from build123d import *

# Parameters (mm, degrees)
SKETCH1_R           = 3.302
BOSS_EXTRUDE1_DEPTH = 6.35
BOSS_EXTRUDE2_START = -6.35
SKETCH2_R           = 3.302
BOSS_EXTRUDE2_DEPTH = 1.5875
BOSS_EXTRUDE3_DEPTH = 12.7
FILLET1_R           = 1.5875
FILLET2_R           = 1.5875


with BuildPart() as part:
    # Sketch1 → Boss-Extrude1 (new body)
    with BuildSketch(Plane.XY):
        with BuildLine():
            Line((10.31875, 31.75), (10.31875, 0))
            ThreePointArc((10.31875, 0), (0, -10.31875), (-10.31875, 0))
            Line((-10.31875, 0), (-10.31875, 31.75))
            ThreePointArc((-10.31875, 31.75), (0, 42.06875), (10.31875, 31.75))
        make_face()
        Circle(SKETCH1_R, mode=Mode.SUBTRACT)
        with Locations((0, 31.75)):
            Circle(SKETCH1_R, mode=Mode.SUBTRACT)
    extrude(amount=BOSS_EXTRUDE1_DEPTH)

    # Sketch2 → Boss-Extrude2 (add)
    with BuildSketch(Plane(origin=(0, 0, 0), x_dir=(-1, 0, 0), z_dir=(0, 0, -1)).offset(BOSS_EXTRUDE2_START)):
        with BuildLine():
            Line((-23.31351417, 8.06700825), (-13.502035234, 36.4220125))
            ThreePointArc((-13.502035234, 36.4220125), (0, 46.0375), (13.502035234, 36.4220125))
            Line((13.502035234, 36.4220125), (23.31351417, 8.06700825))
            ThreePointArc((23.31351417, 8.06700825), (0, -24.66975), (-23.31351417, 8.06700825))
        make_face()
        Circle(SKETCH2_R, mode=Mode.SUBTRACT)
        with Locations((0, 31.75)):
            Circle(SKETCH2_R, mode=Mode.SUBTRACT)
    extrude(amount=BOSS_EXTRUDE2_DEPTH)

    # Sketch3 → Boss-Extrude3 (add)
    with BuildSketch(Plane.XY.offset(6.35)):
        with BuildLine():
            Line((-13.502035234, 36.4220125), (-23.31351417, 8.06700825))
            ThreePointArc((-23.31351417, 8.06700825), (0, -24.66975), (23.31351417, 8.06700825))
            Line((23.31351417, 8.06700825), (13.502035234, 36.4220125))
            ThreePointArc((13.502035234, 36.4220125), (0, 46.0375), (-13.502035234, 36.4220125))
        make_face()
        with BuildLine():
            Line((21.813288033, 7.54789575), (12.001809097, 35.9029))
            ThreePointArc((12.001809097, 35.9029), (0, 44.45), (-12.001809097, 35.9029))
            Line((-12.001809097, 35.9029), (-21.813288033, 7.54789575))
            ThreePointArc((-21.813288033, 7.54789575), (0, -23.08225), (21.813288033, 7.54789575))
        make_face(mode=Mode.SUBTRACT)
    extrude(amount=BOSS_EXTRUDE3_DEPTH)

    # Fillet1
    fillet1_edges = [part.edges().sort_by_distance(p)[0] for p in [
        (10.31875, 15.875, 4.7625),
        (0, 42.06875, 4.7625),
        (-10.31875, 15.875, 4.7625),
        (0, -10.31875, 4.7625),
        (0, 46.0375, 4.7625),
        (18.407774702, 22.244510375, 4.7625),
        (0, -24.66975, 4.7625),
        (-18.407774702, 22.244510375, 4.7625),
        (0, -23.08225, 6.35),
        (16.907548565, 21.725397875, 6.35),
        (0, 44.45, 6.35),
        (-16.907548565, 21.725397875, 6.35),
    ]]
    fillet(fillet1_edges, radius=FILLET1_R)

    # Fillet2
    fillet2_edges = [part.edges().sort_by_distance(p)[0] for p in [
        (10.31875, 15.875, 0),
        (0, -10.31875, 0),
        (-10.31875, 15.875, 0),
        (0, 42.06875, 0),
    ]]
    fillet(fillet2_edges, radius=FILLET2_R)


solid = part.part
Geometry: final body of the model. Coordinates: model frame, mm. A direction names the side the tool comes from. Give positions to 0.01 mm unless a question says otherwise; leave off trailing zeros.
(1) First-contact query: P1, Ø7.5, axis at x = 0, y = 31.75, coming from the +Z side; P2, Ø5.5, axis at x = 0, y = 0, coming from the -Z side; P3, Ø8, axis at x = -10.5, y = 19.5, coming from the -Z side; P4, Ø1.7, axis at y = 16, z = 2.5, coming from the +X side. Flat tips, straight axial feed; report the tip coordinate or a pass-through.
(2) Access query for faces 1 (the cylindrical face through (0.227, -10.316, 2.37)), 2 (the flat face through (10.319, 16, 2)), 3 (the cylindrical face through (17.89, 22.29, 5.22)), 4 (the flat face through (16.976, 21.527, 13.416)). Directions: +Z, -Z, +X, -X, +Y, -Y. A direction counts if a zero-diameter tool reaches every point of the face in a straight line with its end or side. Return the directions, or none.
(3) Ray query, line 1 (Y direction, x = 0, z = 2.25); line 2 (X direction, y = -0.5, z = 17.5); line 3 (Y direction, x = 0, z = 16). Return the intervals inside material, ascending.
(4) Mould query, pull axis Y, two halves, no side actions, for faces 5 (the flat face through (-12, -2, 4.762)), 6 (the flat face through (0, 11, 6.35)), 7 (the flat face through (18.476, 22.046, 12.611)). Classes: released by +Y, released by -Y, zero draft, split by the parting line, or undercut.
(5) Cut plane A-A, the plane x = 0. Give the number of separate pieces and of enclosed holes in the cut face, then the cut area to 3 significant figures.
Values follow:
1. P1: stops at z = 6.35
1. P2: passes through
1. P3: stops at z = 0
1. P4: stops at x = 10.33
2. face 1: -Z, -Y
2. face 2: -Z, +X, +Y, -Y
2. face 3: -Z, +X, +Y
2. face 4: +Z
3. line 1: y = -10.32 to -3.3, 3.3 to 28.45, 35.05 to 42.07
3. line 2: x = -24.66 to -23.08, 23.08 to 24.66
3. line 3: y = -24.67 to -23.08, 44.45 to 46.04
4. face 5: zero draft
4. face 6: undercut
4. face 7: released by +Y
5. separate pieces: 3
5. enclosed holes: 0
5. area: 318 mm2
